The listing builds one solid part. Answer for the finished solid, in the listing's coordinates (mm). Face numbers are marked on the shaded views. A direction names the side the tool comes from. Coordinates: 2 decimals unless noted, no trailing zeros. Order: outer loops, then holes, each group sorted by start corner. A loop starts at its lowest first (then second) coordinate and runs counter-clockwise, first axis right, second up.
Autodesk Inventor part; units mm, degrees
ref_plane "YZ Plane" through (0, 0, 0) normal (1, 0, 0) x (0, 1, 0)
ref_plane "XZ Plane" through (0, 0, 0) normal (0, 1, 0) x (-1, 0, 0)
ref_plane "XY Plane" through (0, 0, 0) normal (0, 0, 1) x (1, 0, 0)
sketch "Boceto1" plane through (0, 0, 0) normal (0, 1, 0) x (-1, 0, 0)
  line L0 (-2.5, 20) -> (2.5, 20)
  line L1 (2.5, 20) -> (2.5, -15)
  line L2 (2.5, -15) -> (-2.5, -15)
  line L3 (-2.5, -15) -> (-2.5, 20)
  line L4 (0, 20) -> (0, -15)
  line L5 (-2.5, 2.5) -> (2.5, 2.5)
  point P0 (0, 0)
  point P1 (0, 2.5)
  dimension "d0" = 5
  dimension "d1" = 35
  dimension "d26" = 20
extrude "Main Body" add sketch "Boceto1" along normal mid plane 100
sketch "Axles" plane through (0, 0, 0) normal (1, 0, 0) x (0, 1, 0)
  line L0 (50, 20) -> (-50, 20)
  circle A0 centre (38, 0) radius 8.05
  circle A1 centre (-40, 0) radius 6.5
  point P0 (0, 0)
  dimension "d53" = 5
  dimension "d55" = 13
  dimension "d11" = 20
  dimension "d12" = 40
  dimension "d13" = 38
  dimension "d14" = 20
  dimension "d22" = 16.1
  dimension "d23" = 13
extrude "Bearings" cut sketch "Axles" along normal mid plane 100
sketch "Boceto4" plane through (0, 0, 0) normal (1, 0, 0) x (0, 1, 0)
  line L0 (-50.2028, -2.5) -> (5.4434, -2.5)
  line L1 (-50, -15) -> (-50, 20)
  line L2 (-50, 7.0921) -> (-15, 7.0921)
  line L3 (-15, 7.0921) -> (-15, -12.9079)
  line L4 (-15, -12.9079) -> (-50, -12.9079)
  line L5 (-50, -12.9079) -> (-50, 7.0921)
  point P0 (0, 0)
  dimension "d27" = 20
  dimension "d28" = 35
sketch "Boceto5" plane through (0, 0, 0) normal (1, 0, 0) x (0, 1, 0)
  line L0 (-50, 25.8088) -> (-15, 25.8088)
  line L1 (-15, 25.8088) -> (-15, -24.1912)
  line L2 (-15, -24.1912) -> (-50, -24.1912)
  line L3 (-50, -24.1912) -> (-50, 25.8088)
  point P0 (0, 0)
  point P1 (-50, 20)
  dimension "d29" = 35
  dimension "d56" = 50
extrude "Spring_support_space" cut sketch "Boceto5" along normal mid plane 10
sketch "Boceto6" plane through (-2.5, -15, 20) normal (0, -1, 0) x (1, 0, 0)
  line L0 (2.5, -16) -> (2.5, -24)
  line L1 (-2.5, -6.5) -> (-2.5, 6.5)
  line L2 (2.5, -20) -> (23.3777, -20)
  line L3 (2.5, 18.3522) -> (2.5, -26.5488)
  circle A0 centre (2.5, -10) radius 1.05
  circle A1 centre (2.5, -30) radius 1.05
  line L4 (0, 0) -> (5, 0)
  line L5 (0, 0) -> (5, 0)
  line L6 (0, -28.05) -> (0, -11.95)
  line L7 (5, -11.95) -> (5, -28.05)
  line L8 (0, -28.05) -> (5, -28.05)
  line L9 (0, -11.95) -> (5, -11.95)
  point P0 (2.5, 0)
  point P1 (0, -20)
  dimension "d35" = 2.1
  dimension "d36" = 20
extrude "Holes" cut sketch "Boceto6" against normal blind 15 contours A0 L3 | L3 A0 | A1
sketch "Boceto10" plane through (-2.5, -15, 20) normal (0, -1, 0) x (1, 0, 0)
  circle A0 centre (2.5, -10) radius 1.05
  circle A1 centre (2.5, -30) radius 1.05
  circle A2 centre (2.5, -10) radius 3.5
  line L0 (-5.1427, -20) -> (9.8665, -20)
  circle A3 centre (2.5, -30) radius 3.5
  point P0 (2.5, -20)
  dimension "d59" = 7
fillet "Edges" radius 15 1 edges at (0, 50, -15)
fillet "Edges" radius 2 1 edges at (0, -15, -15)
sketch "Boceto7" plane through (0, 0, 0) normal (1, 0, 0) x (0, 1, 0)
  line L0 (-15, -15) -> (-15, 20)
  line L1 (-50, 20) -> (50, 20)
  circle A0 centre (-8.5, 17) radius 1.2
  point P0 (0, 0)
  point P1 (45, 20)
  point P2 (-15, 15.1502)
  dimension "d41" = 6.5
  dimension "d42" = 3
  dimension "d50" = 2.4
extrude "Extrusión6" [suppressed]
pattern_linear "Patrón rectangular1" [suppressed]
sketch "Boceto8" plane through (0, 0, 0) normal (1, 0, 0) x (0, 1, 0)
  circle A0 centre (-4.2763, -1.9) radius 1.25
  circle A1 centre (5.7237, -1.9) radius 1.25
  circle A2 centre (15.7237, -1.9) radius 1.25
  point P0 (0, 0)
extrude "Extrusión7" cut sketch "Boceto8" against normal up to surface (5 mm away) from surface at 2.5
sketch "Boceto11" plane through (2.5, -15, 20) normal (1, 0, 0) x (0, 0, -1)
  circle A0 centre (21.9, 10.7237) radius 1.25
  circle A1 centre (21.9, 20.7237) radius 1.25
  circle A2 centre (21.9, 30.7237) radius 1.25
  line L0 (11.05, 0) -> (8.95, 0)
  line L1 (11.05, 15) -> (8.95, 15)
  line L2 (31.05, 0) -> (28.95, 0)
  line L3 (31.05, 15) -> (28.95, 15)
  line L4 (31.05, 0) -> (28.95, 0)
  line L5 (0, 0) -> (33, 0)
  circle A3 centre (20, 53) radius 8.05
  line L6 (0, 65) -> (0, 0)
  line L7 (24.4, 19) -> (26.9, 19)
  line L8 (19.4, 20.9385) -> (19.4, 41.0847)
  line L9 (18.3253, 20) -> (18.3311, 20.0149)
  line L10 (20.4689, 19.9851) -> (20.4635, 20)
  line L11 (19.4, 20.9385) -> (13.1, 38.3464)
  arc A4 (13.1, 42.5769) -> (19.4, 40.5144) centre (20, 53) ccw
  arc A5 (24.4, 41.3) -> (26.9, 42.5769) centre (20, 53) ccw
  line L12 (13.1, 38.3464) -> (13.1, 42.5769)
  line L13 (24.4, 19) -> (24.4, 41.3)
  line L14 (26.9, 19) -> (26.9, 42.5769)
  line L15 (24.4, 19) -> (26.9, 19)
  line L16 (13.1, 4) -> (13.1, 19)
  line L17 (13.1, 34.4694) -> (8, 21)
  line L18 (8, 26.6481) -> (12.0549, 37.3572)
  line L19 (17.9746, 21) -> (13.1, 34.4694)
  line L20 (12.0549, 37.3572) -> (8, 48.5615)
  line L21 (8, 26.6481) -> (8, 48.5615)
  line L22 (13.1, 4) -> (19.4, 4)
  line L23 (24.4, 4) -> (26.9, 4)
  line L24 (24.4, 4) -> (24.4, 19)
  line L25 (26.9, 4) -> (26.9, 19)
  line L26 (19.4, 4) -> (19.4, 19)
  line L27 (13.1, 19) -> (19.4, 19)
  line L28 (8, 21) -> (17.9746, 21)
  point P0 (20, 15)
  point P1 (27.1716, 0)
extrude "Extrusión9" cut sketch "Boceto11" against normal blind 10 contours L13 A5 L14 L7 | L7 L25 L23 L24 | L11 L12 A4 L8 | L16 L27 L26 L22 | L19 L28 L17 | L21 L20 L18
extrude "Extrusión10" [suppressed]
fillet "Empalme2" radius 0.5 18 edges at (0, 6, 2.0254) (0, 19.4694, 6.9) (0, 6, 12) (0, 22.3572, 7.9451) (0, 33.5615, 12) (0, 11.6481, 12) (0, -11, 0.6) (0, 4, 6.9) (0, -11, -6.9) (0, -11, -4.4) (0, 27.5769, -6.9) (0, 26.3, -4.4) (0, 25.5144, 0.6) (0, 27.5769, 6.9) (0, 23.3464, 6.9) (0, 5.9385, 0.6) (0, -11, 6.9) (0, 4, 0.6)
sketch "Boceto13" plane through (-2.5, -15, 20) normal (-1, 0, 0) x (0, 0, 1)
  circle A0 centre (-3, 58.5) radius 1.2
  circle A1 centre (-3, 45.5) radius 1.2
  circle A2 centre (-3, 32.5) radius 1.2
  circle A3 centre (-3, 19.5) radius 1.2
  circle A4 centre (-3, 6.5) radius 1.2
  circle A5 centre (-21.9, 10.7237) radius 1.25
  circle A6 centre (-21.9, 20.7237) radius 1.25
  circle A7 centre (-21.9, 30.7237) radius 1.25
  point P0 (-20, 15)
hole "Agujero4" at (-2.5, -4.2763, -1.9) at (-2.5, 5.7237, -1.9) at (-2.5, 15.7237, -1.9) direction (1, 0, 0) diameter 2.4 end through all countersink diameter 4.6 countersink angle 90
properties part number "support_caterpillar_lateral_v3_Right" material "Plástico ABS"
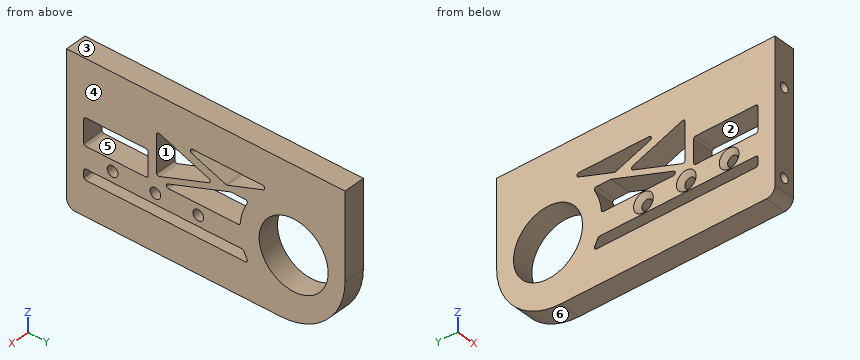
1) Consider L1, parallel to Z at x = -0.05, y = -7; L2, parallel to Z at x = 2.3, y = 2; L3, parallel to X at y = -7, z = 10. Determine where each line is inside the solid, lowest interval first.
2) Section B-B (y = 38) is taken. Give the vertices of the cut face in (x, z), then the cut area to 3 significant figures.
3) Section A-A (z = -1.9) is taken. Give the vertices of the cut face in (x, y), then the cut area to 3 significant figures.
4) Section C-C (z = 10) is taken. Give the vertices of the cut face in (x, y), then the cut area to 3 significant figures.
5) A tool of negligible diameter and unlimited length cuts with its end or side. For the marked faces 5 and 6, from which of +Z, -Z, +X, -X, +Y, -Y can it reach the whole face along a straight path? Write none if from no direction.
6) Determine the mould class of the marked faces 1, 2, 3 and 4 for opening direction Z: released by +Z, released by -Z, zero draft, split by the parting line, or undercut.
7) Each of these flat-tipped pins is pushed along its axis until it touches: P1, Ø1.7, axis at x = -1, z = -5.5, coming from the +Y side; P2, Ø1.7, axis at x = 0, z = 10, coming from the -Y side; P3, Ø3, axis at y = 15.72, z = -1.9, coming from the -X side. Where does it stop, or does it pass through?
8) Section D-D (x = 0) is taken. Give the number of separate pieces and of enclosed holes in the cut face, then the cut area to 3 significant figures.
Filled sheet:
1. L1: z = -15 to -11.05, -8.95 to -6.9, -4.4 to 0.6, 6.9 to 8.95, 11.05 to 20
1. L2: z = -15 to -6.9, -4.4 to 0.6, 6.9 to 20
1. L3: x = -2.5 to -1.05, 1.05 to 2.5
2. outline: (-2.5, -14.7) - (2.5, -14.7) - (2.5, -8.05) - (-2.5, -8.05) - close; (-2.5, 8.05) - (2.5, 8.05) - (2.5, 20) - (-2.5, 20) - close
2. area: 93.0 mm2
3. outline: (-2.5, -15) - (2.5, -15) - (2.5, -5.53) - (-1.45, -5.53) - (-2.5, -6.58) - close; (-2.5, -1.98) - (-1.45, -3.03) - (2.5, -3.03) - (2.5, 4.47) - (-1.45, 4.47) - (-2.5, 3.42) - close; (-2.5, 8.02) - (-1.45, 6.97) - (2.5, 6.97) - (2.5, 14.47) - (-1.45, 14.47) - (-2.5, 13.42) - close; (-2.5, 18.02) - (-1.45, 16.97) - (2.5, 16.97) - (2.5, 30.18) - (-2.5, 30.18) - close; (-2.5, 45.82) - (2.5, 45.82) - (2.5, 49.88) - (-2.5, 49.88) - close
3. area: 205 mm2
4. outline: (-2.5, -15) - (-1.05, -15) - (-1.05, 0) - (1.05, 0) - (1.05, -15) - (2.5, -15) - (2.5, 6) - (-2.5, 6) - close; (-2.5, 11.28) - (2.5, 11.28) - (2.5, 16.93) - (-2.5, 16.93) - close; (-2.5, 28.04) - (2.5, 28.04) - (2.5, 50) - (-2.5, 50) - close
4. area: 212 mm2
5. face 5: +X, -X
5. face 6: -Z, +X, -X, +Y
6. face 1: undercut
6. face 2: undercut
6. face 3: released by +Z
6. face 4: zero draft
7. P1: stops at y = 49.26
7. P2: stops at y = 0
7. P3: stops at x = -1.7
8. separate pieces: 1
8. enclosed holes: 9
8. area: 1,580 mm2
